Geometry check sheet. Reference: the model listing, model coordinates, mm. A direction names the side the tool comes from. Coordinates: 2 decimals unless noted, no trailing zeros. Loops run counter-clockwise (first coordinate to the right, second up) from the corner with the lowest first, then second, coordinate; pieces in that order, holes last. Notation, with made-up numbers: (40.5, 32.25) - (85.5, 32.25) arc R23 cw to (85.5, 44.25) - close; hole circle Ø3 at (-39, 3.5). An arc over 180 degrees is marked (long way). One line per item, written item: value.
from build123d import *

# Parameters (mm, degrees)
SKETCH_1_W          = 8
SKETCH_1_H          = 4
SKETCH_2_R          = 2.1
CUT_EXTRUDE_1_DEPTH = 10
CUT_EXTRUDE_2_DEPTH = 67.588287258


with BuildPart() as part:
    # 草图1 → 旋转1 (revolve)
    with BuildSketch(Plane.XY, mode=Mode.PRIVATE) as revolve_1_sk:
        with Locations((-43, 2)):
            Rectangle(SKETCH_1_W, SKETCH_1_H)
    revolve(revolve_1_sk.sketch.rotate(Axis((0, 0, 0), (0, 1, 0)), 270), axis=Axis((0, 0, 0), (0, 1, 0)))

    # 草图2 → 切除-拉伸1 (cut)
    with BuildSketch(Plane.XZ):
        with Locations(Location((0, 42, 0), (0, 0, 270))):
            Circle(SKETCH_2_R)
        with Locations(Location((29.69848481, 29.69848481, 0), (0, 0, 270))):
            Circle(SKETCH_2_R)
        with Locations(Location((42, 0, 0), (0, 0, 270))):
            Circle(SKETCH_2_R)
        with Locations(Location((29.69848481, -29.69848481, 0), (0, 0, 270))):
            Circle(SKETCH_2_R)
        with Locations(Location((0, -42, 0), (0, 0, 270))):
            Circle(SKETCH_2_R)
        with Locations(Location((-29.69848481, -29.69848481, 0), (0, 0, 270))):
            Circle(SKETCH_2_R)
        with Locations(Location((-42, 0, 0), (0, 0, 270))):
            Circle(SKETCH_2_R)
        with Locations(Location((-29.69848481, 29.69848481, 0), (0, 0, 270))):
            Circle(SKETCH_2_R)
    extrude(amount=-CUT_EXTRUDE_1_DEPTH, mode=Mode.SUBTRACT)

    # 草图3 → 切除-拉伸2 (cut, through all)
    with BuildSketch(Plane(origin=(0, 4, 0), x_dir=(1, 0, 0), z_dir=(0, 1, 0))):
        with BuildLine():
            ThreePointArc((25.237363199, 36.042689949), (16.838071024, 40.65069943), (7.640519817, 43.331541133))
            ThreePointArc((7.640519817, 43.331541133), (5.323607956, 41.709221982), (6.945927107, 39.39231012))
            ThreePointArc((6.945927107, 39.39231012), (15.307337295, 36.9551813), (22.943057454, 32.766081772))
            ThreePointArc((22.943057454, 32.766081772), (25.728514415, 33.257232987), (25.237363199, 36.042689949))
        make_face()
        with BuildLine():
            ThreePointArc((43.331541133, 7.640519817), (40.65069943, 16.838071024), (36.042689949, 25.237363199))
            ThreePointArc((36.042689949, 25.237363199), (33.257232987, 25.728514415), (32.766081772, 22.943057454))
            ThreePointArc((32.766081772, 22.943057454), (36.9551813, 15.307337295), (39.39231012, 6.945927107))
            ThreePointArc((39.39231012, 6.945927107), (41.709221982, 5.323607956), (43.331541133, 7.640519817))
        make_face()
        with BuildLine():
            ThreePointArc((36.042689949, -25.237363199), (40.65069943, -16.838071024), (43.331541133, -7.640519817))
            ThreePointArc((43.331541133, -7.640519817), (41.709221982, -5.323607956), (39.39231012, -6.945927107))
            ThreePointArc((39.39231012, -6.945927107), (36.9551813, -15.307337295), (32.766081772, -22.943057454))
            ThreePointArc((32.766081772, -22.943057454), (33.257232987, -25.728514415), (36.042689949, -25.237363199))
        make_face()
        with BuildLine():
            ThreePointArc((7.640519817, -43.331541133), (16.838071024, -40.65069943), (25.237363199, -36.042689949))
            ThreePointArc((25.237363199, -36.042689949), (25.728514415, -33.257232987), (22.943057454, -32.766081772))
            ThreePointArc((22.943057454, -32.766081772), (15.307337295, -36.9551813), (6.945927107, -39.39231012))
            ThreePointArc((6.945927107, -39.39231012), (5.323607956, -41.709221982), (7.640519817, -43.331541133))
        make_face()
        with BuildLine():
            ThreePointArc((-25.237363199, -36.042689949), (-16.838071024, -40.65069943), (-7.640519817, -43.331541133))
            ThreePointArc((-7.640519817, -43.331541133), (-5.323607956, -41.709221982), (-6.945927107, -39.39231012))
            ThreePointArc((-6.945927107, -39.39231012), (-15.307337295, -36.9551813), (-22.943057454, -32.766081772))
            ThreePointArc((-22.943057454, -32.766081772), (-25.728514415, -33.257232987), (-25.237363199, -36.042689949))
        make_face()
        with BuildLine():
            ThreePointArc((-43.331541133, -7.640519817), (-40.65069943, -16.838071024), (-36.042689949, -25.237363199))
            ThreePointArc((-36.042689949, -25.237363199), (-33.257232987, -25.728514415), (-32.766081772, -22.943057454))
            ThreePointArc((-32.766081772, -22.943057454), (-36.9551813, -15.307337295), (-39.39231012, -6.945927107))
            ThreePointArc((-39.39231012, -6.945927107), (-41.709221982, -5.323607956), (-43.331541133, -7.640519817))
        make_face()
        with BuildLine():
            ThreePointArc((-36.042689949, 25.237363199), (-40.65069943, 16.838071024), (-43.331541133, 7.640519817))
            ThreePointArc((-43.331541133, 7.640519817), (-41.709221982, 5.323607956), (-39.39231012, 6.945927107))
            ThreePointArc((-39.39231012, 6.945927107), (-36.9551813, 15.307337295), (-32.766081772, 22.943057454))
            ThreePointArc((-32.766081772, 22.943057454), (-33.257232987, 25.728514415), (-36.042689949, 25.237363199))
        make_face()
        with BuildLine():
            ThreePointArc((-7.640519817, 43.331541133), (-16.838071024, 40.65069943), (-25.237363199, 36.042689949))
            ThreePointArc((-25.237363199, 36.042689949), (-25.728514415, 33.257232987), (-22.943057454, 32.766081772))
            ThreePointArc((-22.943057454, 32.766081772), (-15.307337295, 36.9551813), (-6.945927107, 39.39231012))
            ThreePointArc((-6.945927107, 39.39231012), (-5.323607956, 41.709221982), (-7.640519817, 43.331541133))
        make_face()
    extrude(amount=-CUT_EXTRUDE_2_DEPTH, mode=Mode.SUBTRACT)


solid = part.part
(1) Material ranges on probe 1 along X at (y, z) = (1.6, 0); probe 2 along Z at (x, y) = (-25, 2.95); probe 3 along X at (y, z) = (0.8, -14), recorded low to high. Write a range as from..to.
Reply:
probe 1: -47..-44.1, -39.9..-39, 39..39.9, 44.1..47
probe 2: -39.8..-36.21, -32.62..-29.93, 29.93..32.62, 36.21..39.8
probe 3: -44.87..-41.71, -37.47..-36.4, 36.4..37.47, 41.71..44.87
(2) Cross-section at B-B on z = 0. Record the cut outline in (x, y).
Reply:
outline: (-47, 0) - (-44.1, 0) - (-44.1, 4) - (-47, 4) - close; (-39.9, 0) - (-39, 0) - (-39, 4) - (-39.9, 4) - close; (39, 0) - (39.9, 0) - (39.9, 4) - (39, 4) - close; (44.1, 0) - (47, 0) - (47, 4) - (44.1, 4) - close
(3) Cross-section at A-A on x = 0. Record the cut outline in (y, z).
Reply:
outline: (0, -47) - (4, -47) - (4, -44.1) - (0, -44.1) - close; (0, -39.9) - (4, -39.9) - (4, -39) - (0, -39) - close; (0, 39) - (4, 39) - (4, 39.9) - (0, 39.9) - close; (0, 44.1) - (4, 44.1) - (4, 47) - (0, 47) - close
(4) Release check for a two-part mould opening along X. For faces 3 (the face through (5.33, 2.03, -41.75)), 4 (the face through (-16.714, 2.028, -40.702)), 5 (the face through (-7, 4, 39)), 6 (the face through (-31.765, 2.028, 34.641)) record: pulls with the +X half, pulls with the -X half, needs draft (parallel to the pull), parting line crosses it, or undercut.
Reply:
face 3: undercut
face 4: undercut
face 5: needs draft
face 6: parting line crosses it
(5) Cross-section at C-C on y = 1.5. State how many separate pieces and enclosed holes the cut face has, and give its area (3 significant figures).
Reply:
separate pieces: 1
enclosed holes: 17
area: 1,360 mm2
(6) Go/stop test with flat-tipped pins: pin 1 Ø2 at (x, y) = (17.5, 2) entering from -Z; pin 2 Ø1 at (y, z) = (1.5, 14.5) entering from -X; pin 3 Ø2 at (y, z) = (1, 22) entering from +X. Record where each tip stops, or that it passes through.
Reply:
pin 1: z = -44.01
pin 2: x = -44.87
pin 3: x = 42.05
(7) Access from +Z, -Z, +X, -X, +Y, -Y to the whole of each face (thin tool, end or side, straight path). Record for faces 1 (the face through (-7, 0, 39)), 2 (the face through (40.6, 2.03, 16.96)).
Reply:
face 1: +Z, -Z, +X, -X, -Y
face 2: +Y, -Y
